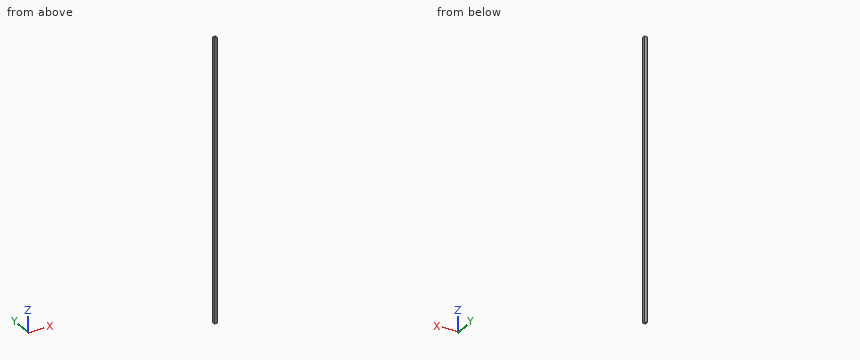
```python
from build123d import *

# Parameters (mm, degrees)
BOSS_EXTRUDE1_DEPTH = 1270


with BuildPart() as part:
    # Sketch1 → Boss-Extrude1 (new body, symmetric)
    with BuildSketch(Plane.XY):
        with BuildLine():
            Line((-11.2903, 13.8303), (11.2903, 13.8303))
            ThreePointArc((11.2903, 13.8303), (13.086351224, 13.086351224), (13.8303, 11.2903))
            Line((13.8303, 11.2903), (13.8303, -11.2903))
            ThreePointArc((13.8303, -11.2903), (13.086351224, -13.086351224), (11.2903, -13.8303))
            Line((11.2903, -13.8303), (-11.2903, -13.8303))
            ThreePointArc((-11.2903, -13.8303), (-13.086351224, -13.086351224), (-13.8303, -11.2903))
            Line((-13.8303, -11.2903), (-13.8303, 11.2903))
            ThreePointArc((-13.8303, 11.2903), (-13.086351224, 13.086351224), (-11.2903, 13.8303))
        make_face()
        with BuildLine():
            Line((-12.5603, 11.2903), (-12.5603, -11.2903))
            ThreePointArc((-12.5603, -11.2903), (-12.188325612, -12.188325612), (-11.2903, -12.5603))
            Line((-11.2903, -12.5603), (11.2903, -12.5603))
            ThreePointArc((11.2903, -12.5603), (12.188325612, -12.188325612), (12.5603, -11.2903))
            Line((12.5603, -11.2903), (12.5603, 11.2903))
            ThreePointArc((12.5603, 11.2903), (12.188325612, 12.188325612), (11.2903, 12.5603))
            Line((11.2903, 12.5603), (-11.2903, 12.5603))
            ThreePointArc((-11.2903, 12.5603), (-12.188325612, 12.188325612), (-12.5603, 11.2903))
        make_face(mode=Mode.SUBTRACT)
    extrude(amount=BOSS_EXTRUDE1_DEPTH, both=True)


solid = part.part
```
Work out the finished part from the listing and answer in its coordinate system (mm). Round coordinates to 2 decimals unless told otherwise and drop trailing zeros. Write each loop counter-clockwise with the first axis right and the second up, starting at its lowest first coordinate (ties: lowest second). Pieces come first, ordered by that corner, then holes. Notation, with made-up numbers: (-28, 20) - (4, 20) arc R10 ccw to (4, 36) - close; hole circle Ø2 at (-1.75, 52.5). An arc over 180 degrees is marked (long way). Return JSON: item names as keys, results as strings. Group by question number.
Q1. The part is cut by section A-A on z = 682. Write down the section's boundary in (x, y), then the cut area to 3 significant figures.
Q2. Find the intervals of material crossed by L1, parallel to X at y = 6.5, z = -1042.5; L2, parallel to X at y = 12.25, z = -785, in increasing order.
Q3. The part is cut by section B-B on y = 0.5. Write down the section's boundary in (x, z).
Solved:
{
 "1": {"outline": "(-13.83, -11.29) arc R2.54 ccw to (-11.29, -13.83) - (11.29, -13.83) arc R2.54 ccw to (13.83, -11.29) - (13.83, 11.29) arc R2.54 ccw to (11.29, 13.83) - (-11.29, 13.83) arc R2.54 ccw to (-13.83, 11.29) - close; hole (-12.56, -11.29) arc R1.27 ccw to (-11.29, -12.56) - (11.29, -12.56) arc R1.27 ccw to (12.56, -11.29) - (12.56, 11.29) arc R1.27 ccw to (11.29, 12.56) - (-11.29, 12.56) arc R1.27 ccw to (-12.56, 11.29) - close", "area": "130 mm²"},
 "2": {"L1": "-13.83 to -12.56, 12.56 to 13.83", "L2": "-13.64 to -12.12, 12.12 to 13.64"},
 "3": {"outline": "(-13.83, -1270) - (-12.56, -1270) - (-12.56, 1270) - (-13.83, 1270) - close; (12.56, -1270) - (13.83, -1270) - (13.83, 1270) - (12.56, 1270) - close"}
}
